```python
from build123d import *

# Parameters (mm, degrees)
EXTRUDE_1_DEPTH     = 50
SKETCH_2_R          = 1.75
CUT_EXTRUDE_1_DEPTH = 85.787970845
CUT_EXTRUDE_3_REACH = 86.788
SKETCH_4_R          = 1.75
SKETCH_4_R_2        = 2.25


with BuildPart() as part:
    # 草图1 → 凸台-拉伸1 (new body)
    with BuildSketch(Plane(origin=(0, 0, 0), x_dir=(1, 0, 0), z_dir=(0, 1, 0))):
        Polygon((0, 0), (30, 0), (30, 60), (33, 60), (33, -3), (0, -3), align=None)
    extrude(amount=EXTRUDE_1_DEPTH)

    # 草图2 → 切除-拉伸1 (cut, through all)
    with BuildSketch(Plane(origin=(0, 0, 0), x_dir=(-1, 0, 0), z_dir=(0, 0, -1))):
        with Locations((-22, 6)):
            Circle(SKETCH_2_R)
        with Locations((-22, 44)):
            Circle(SKETCH_2_R)
        with Locations((-5, 44)):
            Circle(SKETCH_2_R)
        with Locations((-5, 6)):
            Circle(SKETCH_2_R)
    extrude(amount=-CUT_EXTRUDE_1_DEPTH, mode=Mode.SUBTRACT)

    # 草图4 → 切除-拉伸3 (cut, up to next)
    with BuildSketch(Plane(origin=(33, 0, 0), x_dir=(0, 0, -1), z_dir=(1, 0, 0)), mode=Mode.PRIVATE) as cut_extrude_3_sk1:
        with Locations((56.5, 25)):
            Circle(SKETCH_4_R)
    cut_extrude_3_tool1 = extrude(cut_extrude_3_sk1.sketch, amount=-CUT_EXTRUDE_3_REACH, mode=Mode.PRIVATE) & part.part
    # 草图4 → 切除-拉伸3 (cut, up to next)
    with BuildSketch(Plane(origin=(33, 0, 0), x_dir=(0, 0, -1), z_dir=(1, 0, 0)), mode=Mode.PRIVATE) as cut_extrude_3_sk2:
        with Locations((31.5, 25)):
            Circle(SKETCH_4_R)
    cut_extrude_3_tool2 = extrude(cut_extrude_3_sk2.sketch, amount=-CUT_EXTRUDE_3_REACH, mode=Mode.PRIVATE) & part.part
    # 草图4 → 切除-拉伸3 (cut, up to next)
    with BuildSketch(Plane(origin=(33, 0, 0), x_dir=(0, 0, -1), z_dir=(1, 0, 0)), mode=Mode.PRIVATE) as cut_extrude_3_sk3:
        with Locations((22, 46)):
            Circle(SKETCH_4_R_2)
    cut_extrude_3_tool3 = extrude(cut_extrude_3_sk3.sketch, amount=-CUT_EXTRUDE_3_REACH, mode=Mode.PRIVATE) & part.part
    # 草图4 → 切除-拉伸3 (cut, up to next)
    with BuildSketch(Plane(origin=(33, 0, 0), x_dir=(0, 0, -1), z_dir=(1, 0, 0)), mode=Mode.PRIVATE) as cut_extrude_3_sk4:
        with Locations((22, 4)):
            Circle(SKETCH_4_R_2)
    cut_extrude_3_tool4 = extrude(cut_extrude_3_sk4.sketch, amount=-CUT_EXTRUDE_3_REACH, mode=Mode.PRIVATE) & part.part
    add(cut_extrude_3_tool1.solids().sort_by_distance((33, 25, -56.5))[0], mode=Mode.SUBTRACT)
    add(cut_extrude_3_tool2.solids().sort_by_distance((33, 25, -31.5))[0], mode=Mode.SUBTRACT)
    add(cut_extrude_3_tool3.solids().sort_by_distance((33, 46, -22))[0], mode=Mode.SUBTRACT)
    add(cut_extrude_3_tool4.solids().sort_by_distance((33, 4, -22))[0], mode=Mode.SUBTRACT)


solid = part.part
```
Input: part model. Units: mm. Frame: model coordinates. A direction names the side the tool comes from. Give positions to 0.01 mm unless a question says otherwise; leave off trailing zeros. Order: outer loops, then holes, each group sorted by start corner. A loop starts at its lowest first (then second) coordinate and runs counter-clockwise, first axis right, second up.
1. Pin query (flat end, axial travel): pin 1 (3 mm diameter, centred on y = 44, z = -11.5, fed in from -X); pin 2 (4.5 mm diameter, centred on x = 5, y = 44, fed in from -Z). Return the tip coordinate at first contact, or that it passes through.
Derived:
pin 1: stops at x = 30
pin 2: stops at z = 0
2. Section A-A on y = 25. Return the cut outline in (x, z).
Derived:
outline: (0, 0) - (30, 0) - (30, -29.75) - (33, -29.75) - (33, 3) - (0, 3) - close; (30, -60) - (33, -60) - (33, -58.25) - (30, -58.25) - close; (30, -54.75) - (33, -54.75) - (33, -33.25) - (30, -33.25) - close
3. Material intervals for L1, parallel to Y at x = 22, z = 2.3; L2, parallel to Y at x = 31.9, z = -22; L3, parallel to Y at x = 32.35, z = -56.5, sorted ascending.
Derived:
L1: y = 0 to 4.25, 7.75 to 42.25, 45.75 to 50
L2: y = 0 to 1.75, 6.25 to 43.75, 48.25 to 50
L3: y = 0 to 23.25, 26.75 to 50
4. Mould query, pull axis Y, two halves, no side actions, for faces 1 (the flat face through (31, 0, -22)), 2 (the flat face through (33, 25, -29)), 3 (the cylindrical face through (31.521, 47.897, -23.21)). Classes: released by +Y, released by -Y, zero draft, split by the parting line, or undercut.
Derived:
face 1: released by -Y
face 2: zero draft
face 3: undercut
5. Section C-C on z = -22. Return the cut outline in (x, y), and give its area (3 significant figures).
Derived:
outline: (30, 0) - (33, 0) - (33, 1.75) - (30, 1.75) - close; (30, 6.25) - (33, 6.25) - (33, 43.75) - (30, 43.75) - close; (30, 48.25) - (33, 48.25) - (33, 50) - (30, 50) - close
area: 123 mm2
6. Section B-B on x = 5. Return the cut outline in (y, z).
Derived:
outline: (0, 0) - (4.25, 0) - (4.25, 3) - (0, 3) - close; (7.75, 0) - (42.25, 0) - (42.25, 3) - (7.75, 3) - close; (45.75, 0) - (50, 0) - (50, 3) - (45.75, 3) - close
7. Reachability of faces 4 (the flat face through (31, 50, -22)), 5 (the flat face through (15, 25, 0)) from +Z, -Z, +X, -X, +Y, -Y: full face, straight path, thin tool, end or side. Return the list, or none.
Derived:
face 4: +Z, -Z, +X, -X, +Y
face 5: -Z, -X, +Y, -Y
8. Section D-D on y = 31.5. Return the cut outline in (x, z).
Derived:
outline: (0, 0) - (30, 0) - (30, -60) - (33, -60) - (33, 3) - (0, 3) - close
